from build123d import *

# Parameters (mm, degrees)
PAD001_DEPTH  = 3
SKETCH014_R   = 2.000997
SKETCH014_R_2 = 1.989716
SKETCH014_R_3 = 2.044982
SKETCH014_R_4 = 1.975414
SKETCH014_R_5 = 2.027461
SKETCH014_R_6 = 1.954742
SKETCH014_R_7 = 2.009119
PAD013_DEPTH  = 2
SKETCH015_R   = 2
POCKET_DEPTH  = 2


with BuildPart() as part:
    # Sketch002 → Pad001 (new body)
    with BuildSketch(Plane.XY):
        with BuildLine():
            Line((158.170695, -17.490656), (158.170695, -16.535702))
            ThreePointArc((160.837743, -13.868068), (158.954121, -14.651909), (158.170695, -16.535702))
            Line((161.975632, -13.868068), (160.837743, -13.868068))
            Line((161.975632, -13.868068), (214.050903, -13.868068))
            ThreePointArc((214.050903, -13.868068), (214.951659, -13.498902), (215.320954, -12.598198))
            Line((215.320954, -12.598198), (215.320954, -12.216596))
            ThreePointArc((216.59103, -10.947382), (215.694908, -11.320728), (215.320954, -12.216596))
            Line((216.59103, -10.947382), (218.273682, -10.947382))
            Line((218.273682, -10.947382), (233.355242, -10.947382))
            ThreePointArc((234.625102, -12.21752), (234.252072, -11.320608), (233.355242, -10.947382))
            Line((234.625102, -12.21752), (234.625102, -12.598559))
            ThreePointArc((234.625102, -12.598559), (234.994142, -13.499389), (235.895, -13.868359))
            Line((235.895, -13.868359), (238.271805, -13.868359))
            Line((238.271805, -13.868359), (252.40531, -13.868359))
            ThreePointArc((253.674886, -15.138264), (253.301131, -14.242347), (252.40531, -13.868359))
            Line((253.674886, -15.138264), (253.674886, -16.154515))
            ThreePointArc((253.674886, -16.154515), (254.046325, -17.05216), (254.943533, -17.424653))
            Line((254.943533, -17.424653), (298.758985, -17.424653))
            ThreePointArc((301.426813, -20.093175), (300.642993, -18.208962), (298.758985, -17.424653))
            Line((301.426813, -20.093175), (301.426813, -110.261392))
            ThreePointArc((298.759763, -112.928087), (300.646389, -112.147914), (301.426813, -110.261392))
            Line((298.759763, -112.928087), (296.766937, -112.928087))
            Line((296.766937, -112.928087), (254.690998, -112.928087))
            ThreePointArc((253.420935, -111.658351), (253.793197, -112.556056), (254.690998, -112.928087))
            Line((253.420935, -111.658351), (253.420935, -110.642303))
            ThreePointArc((253.420935, -110.642303), (253.045275, -109.745808), (252.147799, -109.372497))
            Line((252.147799, -109.372497), (196.525526, -109.372497))
            ThreePointArc((196.525526, -109.372497), (195.461836, -109.538225), (194.493223, -110.008001))
            ThreePointArc((194.493223, -110.008001), (180.053907, -119.312238), (167.31519, -130.835593))
            ThreePointArc((165.282705, -130.835445), (166.298917, -131.255159), (167.31519, -130.835593))
            Line((165.282705, -130.835445), (153.598862, -119.151413))
            ThreePointArc((153.598907, -117.119461), (153.178634, -118.135428), (153.598862, -119.151413))
            Line((153.598907, -117.119461), (157.024855, -113.694223))
            ThreePointArc((157.024855, -113.694223), (158.518785, -107.850658), (157.027893, -102.006317))
            Line((157.027893, -102.006317), (158.170695, -95.78363))
            Line((158.170695, -95.78363), (158.170695, -17.490656))
        make_face()
    extrude(amount=-PAD001_DEPTH)

    # Sketch014 → Pad013 (join)
    with BuildSketch(Plane.XY):
        with Locations((253.550873, -34.889503)):
            Circle(SKETCH014_R)
        with Locations((253.5784, -91.939972)):
            Circle(SKETCH014_R_2)
        with Locations((196.387711, -72.36747)):
            Circle(SKETCH014_R_3)
        with Locations((215.512299, -31.736803)):
            Circle(SKETCH014_R_4)
        with Locations((215.534556, -88.769968)):
            Circle(SKETCH014_R_5)
        with Locations((234.534821, -69.803696)):
            Circle(SKETCH014_R_6)
        with Locations((234.538681, -50.705391)):
            Circle(SKETCH014_R_7)
        with Locations((183.832245, -35.004906)):
            Circle(SKETCH014_R_4)
    extrude(amount=PAD013_DEPTH)

    # Sketch015 (on Face37 of Pad001) → Pocket (cut)
    with BuildSketch(Plane.XY):
        with Locations((166.298927, -128.044507)):
            Circle(SKETCH015_R)
        with Locations((297.965025, -109.472203)):
            Circle(SKETCH015_R)
        with Locations((160.45478, -19.71329)):
            Circle(SKETCH015_R)
        with Locations((297.96712, -20.569173)):
            Circle(SKETCH015_R)
        with Locations((162.270263, -105.690893)):
            Circle(SKETCH015_R)
    extrude(amount=-POCKET_DEPTH, mode=Mode.SUBTRACT)


solid = part.part
CAD build for the part. Positions are in the model's coordinates, mm. A direction names the side the tool comes from. Give positions to 0.01 mm unless a question says otherwise; leave off trailing zeros. Order: outer loops, then holes, each group sorted by start corner. A loop starts at its lowest first (then second) coordinate and runs counter-clockwise, first axis right, second up. Notation, with made-up numbers: (51.25, 53.5) -> (61.25, 53.5) arc R16 cw to (61.25, 63.5) -> close; hole circle Ø8 at (55, -20). An arc over 180 degrees is marked (long way). Return JSON: item names as keys, results as strings.
Q1. Saw through at B-B (x = 264). Write the cut outline in (y, z).
Working result:
{"outline": "(-112.93, -3) -> (-17.42, -3) -> (-17.42, 0) -> (-112.93, 0) -> close"}
Q2. Saw through at C-C (y = -24.5). Write the cut outline in (x, z), then the cut area to 3 significant figures.
Working result:
{"outline": "(158.17, -3) -> (301.43, -3) -> (301.43, 0) -> (158.17, 0) -> close", "area": "430 mm²"}
Q3. Drill centre lines: line 1 (X direction, y = -21.5, z = -0.75); line 2 (X direction, y = -109, z = -2.2); line 3 (Z direction, x = 177, y = -65.5). Where is each one in solid material? Low to high.
Working result:
{"line 1": "158.17 to 159.56, 161.35 to 296.2, 299.74 to 301.43", "line 2": "158.46 to 301.43", "line 3": "-3 to 0"}
Q4. Flat gauge pins, fed straight in: pin 1 (0.5 mm diameter, centred on y = -111, z = -1.5, fed in from -X); pin 2 (1.2 mm diameter, centred on x = 298.5, y = -21, fed in from +Z); pin 3 (1.5 mm diameter, centred on x = 284, z = -2, fed in from +Y). Where does each tip first touch, or does it go through?
Working result:
{"pin 1": "x = 158.03", "pin 2": "z = -2", "pin 3": "y = -17.42"}
Q5. Mould opens along Y. For faces 5 (the face through (225, -10.947, -1)), 6 (the face through (225, -109.372, -1)), 7 (the face through (158.52, -107.94, -1.48)) say: pulls with the +Y half, pulls with the -Y half, needs draft (parallel to the pull), parting line crosses it, or undercut.
Working result:
{"face 5": "pulls with the +Y half", "face 6": "pulls with the -Y half", "face 7": "undercut"}
Q6. Saw through at A-A (z = 0.9). Write the cut outline in (x, y).
Working result:
{"outline": "circle Ø3.95 at (183.83, -35); circle Ø4.09 at (196.39, -72.37); circle Ø4.05 at (215.53, -88.77); circle Ø3.95 at (215.51, -31.74); circle Ø4.02 at (234.54, -50.71); circle Ø3.91 at (234.53, -69.8); circle Ø4 at (253.55, -34.89); circle Ø3.98 at (253.58, -91.94)"}
Q7. Which spindle directions (+Z, -Z, +X, -X, +Y, -Y) get a long thin tool onto all of the face, cutting with end or side? Do faces 1 (the face through (236.455, -50.102, 0.986)), 2 (the face through (180.2, -119.2, -1.5)), 3 (the face through (277, -112.928, -1)), 4 (the face through (158.171, -57, -1)). Say none if no direction does.
Working result:
{"face 1": "+Z", "face 2": "+Z, -Z, -Y", "face 3": "+Z, -Z, +X, -Y", "face 4": "+Z, -Z, -X, +Y"}
